Could you check a few things on this drawing? It's one solid part, dimensions in mm from its lowest x, y, z. Give positions to 0.01 mm unless a question says otherwise; leave off trailing zeros. Loops run counter-clockwise (first coordinate to the right, second up) from the corner with the lowest first, then second, coordinate; pieces in that order, holes last. Notation, with made-up numbers: M 67,86 L 123,86 A19 ccw 123,114 Z; hole C -39.5,-13 d3. An arc over 180 degrees is marked long. Return JSON: item names as keys, results as strings. Group by question number.
1. For pin 1 (3.5 mm diameter, centred on x = 6.5, z = 6.5, fed in from +Y), with a flat end and sliding along its axis, tell me the tip position at first contact or that it passes through.
2. If we section it at B-B (x = 6.5): Write out the boundary of the cut face in (y, z), plus the area to 3 significant figures.
3. Please list where these lines run through material, in increasing order: line 1 (X direction, y = 2, z = 6.5); line 2 (Z direction, x = 4, y = 1.4); line 3 (X direction, y = 0.7, z = 8).
4. If we section it at A-A (z = 6.5): Write out the boundary of the cut face in (x, y).
5. If we mould it in two halves opening along X, with no side actions, what happens to the marked faces 1, 2 and 3? For each: +X half, -X half, draft (parallel to the pull), parting line (faces both ways), or undercut.
6. If we section it at C-C (y = 1.7): Write out the boundary of the cut face in (x, z), plus the area to 3 significant figures.
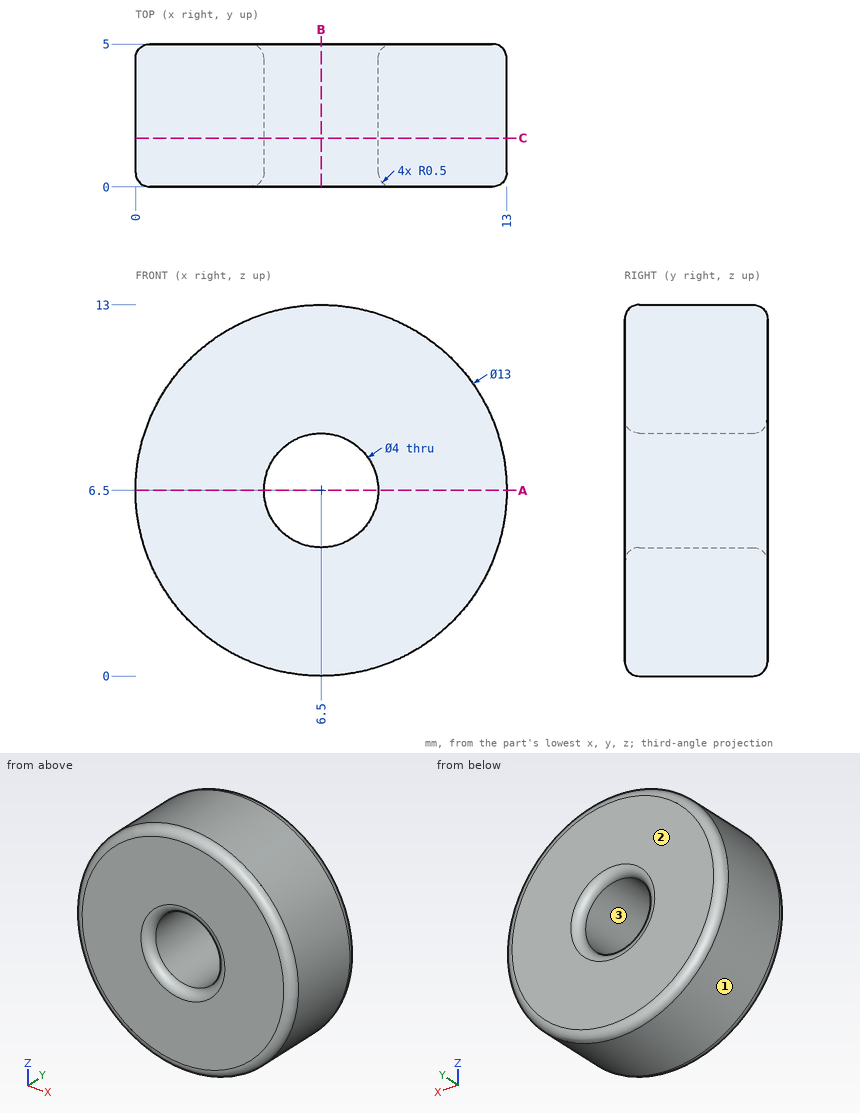
Answer:
{
 "1": {"pin 1": "passes through"},
 "2": {"outline": "M 0,0.5 A0.5 ccw 0.5,0 L 4.5,0 A0.5 ccw 5,0.5 L 5,4 A0.5 ccw 4.5,4.5 L 0.5,4.5 A0.5 ccw 0,4 Z; M 0,9 A0.5 ccw 0.5,8.5 L 4.5,8.5 A0.5 ccw 5,9 L 5,12.5 A0.5 ccw 4.5,13 L 0.5,13 A0.5 ccw 0,12.5 Z", "area": "44.6 mm²"},
 "3": {"line 1": "x = 0 to 4.5, 8.5 to 13", "line 2": "z = 0.5 to 12.5", "line 3": "x = 0.18 to 5.18, 7.82 to 12.82"},
 "4": {"outline": "M 0,0.5 A0.5 ccw 0.5,0 L 4,0 A0.5 ccw 4.5,0.5 L 4.5,4.5 A0.5 ccw 4,5 L 0.5,5 A0.5 ccw 0,4.5 Z; M 8.5,0.5 A0.5 ccw 9,0 L 12.5,0 A0.5 ccw 13,0.5 L 13,4.5 A0.5 ccw 12.5,5 L 9,5 A0.5 ccw 8.5,4.5 Z"},
 "5": {"face 1": "parting line", "face 2": "draft", "face 3": "undercut"},
 "6": {"outline": "C 6.5,6.5 d13; hole C 6.5,6.5 d4", "area": "120 mm²"}
}
